Could you check a few things on this model? Use its own coordinates, in mm. Face numbers are marked on the shaded views. A direction names the side the tool comes from. Give positions to 0.01 mm unless a question says otherwise; leave off trailing zeros. Loops run counter-clockwise (first coordinate to the right, second up) from the corner with the lowest first, then second, coordinate; pieces in that order, holes last. Notation, with made-up numbers: (21.5, 59.25) - (69.5, 59.25) arc R22 cw to (69.5, 65.25) - close; hole circle Ø2 at (88, 14.25). An arc over 180 degrees is marked (long way). Write each question's results on one line, items separated by ' | '. Start each with the question number.
```python
from build123d import *

# Parameters (mm, degrees)
SKETCH_1_R          = 15
EXTRUDE_1_DEPTH     = 17
SKETCH_2_R          = 11
EXTRUDE_2_DEPTH     = 1.5
SKETCH_3_R          = 15
EXTRUDE_3_DEPTH     = 3
SKETCH_4_R          = 11
EXTRUDE_4_DEPTH     = 4.5
SKETCH_6_W          = 44
SKETCH_6_H          = 30
EXTRUDE_6_DEPTH     = 52
SKETCH_7_W          = 5
SKETCH_7_H          = 30
EXTRUDE_7_DEPTH     = 2
SKETCH_8_W          = 22
SKETCH_8_H          = 20
CUT_EXTRUDE_1_DEPTH = 87.417590802
SKETCH_9_R          = 13
SKETCH_9_R_2        = 12
CUT_EXTRUDE_2_DEPTH = 2


with BuildPart() as part:
    # 草圖1 → 伸長1 (new body)
    with BuildSketch(Plane(origin=(0, 0, 0), x_dir=(1, 0, 0), z_dir=(0, 1, 0))):
        with Locations(Location((0, 0, 0), (0, 0, 270))):
            Circle(SKETCH_1_R)
    extrude(amount=EXTRUDE_1_DEPTH)

    # 草圖2 → 伸長2 (add)
    with BuildSketch(Plane(origin=(0, 17, 0), x_dir=(1, 0, 0), z_dir=(0, 1, 0))):
        with Locations(Location((0, 0, 0), (0, 0, 270))):
            Circle(SKETCH_2_R)
    extrude(amount=EXTRUDE_2_DEPTH)

    # 草圖3 → 伸長3 (add)
    with BuildSketch(Plane(origin=(0, 18.5, 0), x_dir=(1, 0, 0), z_dir=(0, 1, 0))):
        with Locations(Location((0, 0, 0), (0, 0, 270))):
            Circle(SKETCH_3_R)
    extrude(amount=EXTRUDE_3_DEPTH)

    # 草圖4 → 伸長4 (add)
    with BuildSketch(Plane(origin=(0, 21.5, 0), x_dir=(1, 0, 0), z_dir=(0, 1, 0))):
        with Locations(Location((0, 0, 0), (0, 0, 270))):
            Circle(SKETCH_4_R)
    extrude(amount=EXTRUDE_4_DEPTH)

    # 草圖6 → 伸長6 (add)
    with BuildSketch(Plane(origin=(0, 26, 0), x_dir=(1, 0, 0), z_dir=(0, 1, 0))):
        Rectangle(SKETCH_6_W, SKETCH_6_H)
    extrude(amount=EXTRUDE_6_DEPTH)

    # 草圖7 → 伸長7 (add)
    with BuildSketch(Plane.XZ.offset(-26)):
        with Locations((-19.5, 0)):
            Rectangle(SKETCH_7_W, SKETCH_7_H)
    extrude(amount=EXTRUDE_7_DEPTH)

    # 草圖8 → 除料-伸長1 (cut, through all)
    with BuildSketch(Plane(origin=(0, 0, -15), x_dir=(-1, 0, 0), z_dir=(0, 0, -1))):
        with Locations((11, 68)):
            Rectangle(SKETCH_8_W, SKETCH_8_H)
    extrude(amount=-CUT_EXTRUDE_1_DEPTH, mode=Mode.SUBTRACT)

    # 草圖9 → 除料-伸長2 (cut)
    with BuildSketch(Plane.XZ):
        with Locations(Location((0, 0, 0), (0, 0, 270))):
            Circle(SKETCH_9_R)
        with Locations(Location((0, 0, 0), (0, 0, 270))):
            Circle(SKETCH_9_R_2, mode=Mode.SUBTRACT)
    extrude(amount=-CUT_EXTRUDE_2_DEPTH, mode=Mode.SUBTRACT)


solid = part.part
```
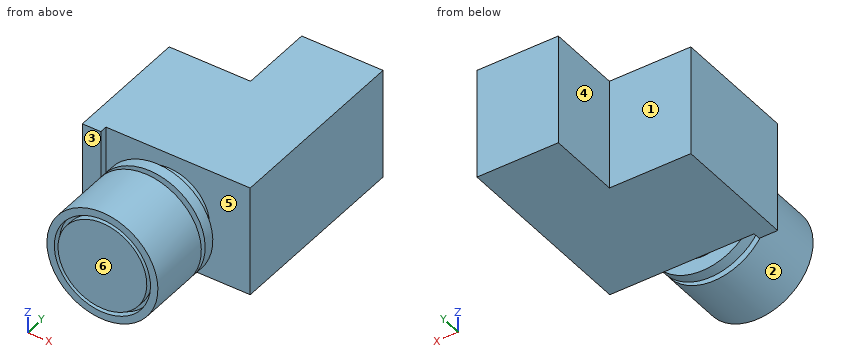
Q1. I need wall thicknesses on L1, parallel to X at y = 0.7, z = 0; L2, parallel to Y at x = 11, z = -9.25; L3, parallel to Y at x = -2, z = 11.5. Which ranges of each line are inside material? Lowest first, please. Write a range as from..to.
Q2. I'm going to push flat-ended pins straight in: pin 1 Ø17.5 at (x, z) = (-14, 1.5) entering from +Y; pin 2 Ø10 at (y, z) = (11, 1.5) entering from +X; pin 3 Ø5 at (y, z) = (20.5, 8) entering from -X. Where does each tip first touch, or does it pass through?
Q3. I want a section at C-C, the plane x = 19.5. List the corners of the cut face in (y, z) for me, then the cut area to 3 significant figures.
Q4. I want a section at B-B, the plane y = 16. List the corners of the cut face in (x, z) for me, then the cut area to 3 significant figures.
Q5. If we mould it in two halves opening along Y, with no side actions, what happens to the marked faces 4, 5 and 6? For each: +Y half, -Y half, draft (parallel to the pull), parting line (faces both ways), or undercut.
Q6. Which directions (+Z, -Z, +X, -X, +Y, -Y) give clear straight access to the entire face, cutting with the end or side of a thin tool? Please do the marked faces 1, 2 and 3.
Conclusion:
1) L1: -15..-13, -12..12, 13..15 | L2: 0..17, 18.5..21.5, 26..78 | L3: 0..17, 18.5..21.5, 26..58
2) pin 1: y = 58 | pin 2: x = 15 | pin 3: x = -13.96
3) outline: (26, -15) - (78, -15) - (78, 15) - (26, 15) - close | area: 1,560 mm^2
4) outline: circle Ø30 at (0, 0) | area: 707 mm^2
5) face 4: draft | face 5: undercut | face 6: -Y half
6) face 1: +Z, -Z, -X, +Y | face 2: -Y | face 3: +Z, -Z, -X, -Y
